Model file for the job. Use its own axes, mm. A direction names the side the tool comes from. Round coordinates to 2 decimals unless told otherwise and drop trailing zeros. Order: outer loops, then holes, each group sorted by start corner. A loop starts at its lowest first (then second) coordinate and runs counter-clockwise, first axis right, second up. Notation, with made-up numbers: (64.5, -1.5) - (92.5, -1.5) arc R25 ccw to (92.5, 23.5) - close; hole circle Ø3 at (71, 29.25). An arc over 180 degrees is marked (long way). Answer as CSV lines item,"result". Start each with the question number.
1. Band-saw the part on D-D on y = 10.75. List the corners of the cut face in (x, z), then the cut area to 3 significant figures.
2. Band-saw the part on A-A on x = 0. List the corners of the cut face in (y, z).
3. Band-saw the part on C-C on x = -26. List the corners of the cut face in (y, z).
4. 3-axis set-ups, long thin cutter, end or side, ignore diameter. For faces 5 (the face through (2, 16.764, -3)), 6 (the face through (3.399, 0.505, -15.933)), 7 (the face through (2, 0, 4)): which of +Z, -Z, +X, -X, +Y, -Y reach the whole face in a straight line?
5. Wall check: line 1 along Z through (x, y) = (0, -3.75); line 2 along Z through (x, y) = (0, 2.75); line 3 along X through (y, z) = (-5, -8.75). Give the ranges that are in metal, low to high. Write a range as [from, to].
6. Pin check, flat tips, straight feed: pin 1 Ø3 at (x, z) = (14.5, 4) entering from -Y; pin 2 Ø2 at (x, z) = (5, -11) entering from -Y; pin 3 Ø4 at (x, y) = (-6, -6) entering from +Z. Stop position of each tip, or through.
7. Pull direction Z, two halves, no side cores. Call faces 1 (the face through (2.311, -0.724, 0.764)), 2 (the face through (-21.57, 4.24, -10.92)), 3 (the face through (2, 4, -19.05)), 4 (the face through (-36.322, 4, -7)): released by +Z, released by -Z, zero draft, split by the parting line, or undercut.
8. Band-saw the part on B-B on z = -6.25. List the corners of the cut face in (x, y), then the cut area to 3 significant figures.
```python
from build123d import *

# Parameters (mm, degrees)
BOSS_EXTRUDE1_DEPTH      = 39.878
BOSS_EXTRUDE1_DEPTH_BACK = 36.322
FILLET1_R                = 2.54
SKETCH2_R                = 5.08
SKETCH2_R_2              = 5.842
CUT_EXTRUDE1_DEPTH       = 26.4
SKETCH3_R                = 7.366
CUT_EXTRUDE2_DEPTH       = 18.542


with BuildPart() as part:
    # Sketch1 → Boss-Extrude1 (new body, two sides)
    with BuildSketch(Plane(origin=(0, 0, 0), x_dir=(0, 0, -1), z_dir=(1, 0, 0))) as boss_extrude1_sk:
        Polygon((0, 0), (-6.35, 0), (-6.35, 16.764), (19.05, 16.764), (19.05, -8.636), (0, -8.636), align=None)
    extrude(amount=BOSS_EXTRUDE1_DEPTH)
    extrude(boss_extrude1_sk.sketch, amount=-BOSS_EXTRUDE1_DEPTH_BACK)

    # Fillet1
    fillet1_edges = [part.edges().sort_by_distance(p)[0] for p in [
        (1.778, 0, 0),
    ]]
    fillet(fillet1_edges, radius=FILLET1_R)

    # Sketch2 → Cut-Extrude1 (cut, through all)
    with BuildSketch(Plane(origin=(0, 16.764, 0), x_dir=(1, 0, 0), z_dir=(0, 1, 0))):
        with Locations((-26.416, 9.398)):
            Circle(SKETCH2_R)
        with Locations((32.258, 9.398)):
            Circle(SKETCH2_R)
        with Locations((0, 9.398)):
            Circle(SKETCH2_R_2)
    extrude(amount=-CUT_EXTRUDE1_DEPTH, mode=Mode.SUBTRACT)

    # Sketch3 → Cut-Extrude2 (cut)
    with BuildSketch(Plane.XZ.offset(8.636)):
        with Locations((0, -9.398)):
            Circle(SKETCH3_R)
    extrude(amount=-CUT_EXTRUDE2_DEPTH, mode=Mode.SUBTRACT)


solid = part.part
```
Reply:
1,outline,"(-36.32, -19.05) - (39.88, -19.05) - (39.88, 6.35) - (-36.32, 6.35) - close; hole circle Ø10.16 at (-26.42, -9.4); hole circle Ø11.68 at (0, -9.4); hole circle Ø10.16 at (32.26, -9.4)"
1,area,"1,670 mm2"
2,outline,"(-8.64, -19.05) - (16.76, -19.05) - (16.76, -15.24) - (9.91, -15.24) - (9.91, -16.76) - (-8.64, -16.76) - close; (-8.64, -2.03) - (9.91, -2.03) - (9.91, -3.56) - (16.76, -3.56) - (16.76, 6.35) - (0, 6.35) - (0, 2.54) arc R2.54 cw to (-2.54, 0) - (-8.64, 0) - close"
3,outline,"(-8.64, -19.05) - (16.76, -19.05) - (16.76, -14.46) - (-8.64, -14.46) - close; (-8.64, -4.34) - (16.76, -4.34) - (16.76, 6.35) - (0, 6.35) - (0, 2.54) arc R2.54 cw to (-2.54, 0) - (-8.64, 0) - close"
4,face 5,"+Z, -Z, +X, -X, +Y"
4,face 6,"-Y"
4,face 7,"+Z, +X, -X, -Y"
5,line 1,"z = [-19.05, -16.76], [-2.03, 0]"
5,line 2,"z = [-19.05, -16.76], [-2.03, 6.35]"
5,line 3,"x = [-36.32, -31.45], [-21.38, -7.34], [7.34, 27.22], [37.3, 39.88]"
6,pin 1,"stops at y = 0"
6,pin 2,"stops at y = 9.91"
6,pin 3,"stops at z = 0"
7,face 1,"released by +Z"
7,face 2,"undercut"
7,face 3,"released by -Z"
7,face 4,"zero draft"
8,outline,"(-36.32, -8.64) - (-30.4, -8.64) - (-30.4, 16.76) - (-36.32, 16.76) - close; (-22.43, -8.64) - (-6.66, -8.64) - (-6.66, 9.91) - (-4.92, 9.91) - (-4.92, 16.76) - (-22.43, 16.76) - close; (4.92, 9.91) - (6.66, 9.91) - (6.66, -8.64) - (28.27, -8.64) - (28.27, 16.76) - (4.92, 16.76) - close; (36.25, -8.64) - (39.88, -8.64) - (39.88, 16.76) - (36.25, 16.76) - close"
8,area,"1,220 mm2"
